Input: part model. Units: mm. Frame: model coordinates. A direction names the side the tool comes from. Coordinates: 2 decimals unless noted, no trailing zeros. Loops run counter-clockwise (first coordinate to the right, second up) from the corner with the lowest first, then second, coordinate; pieces in that order, holes last. Notation, with made-up numbers: (64, -15.5) -> (97, -15.5) arc R22 ccw to (97, 23.5) -> close; hole circle Ø9 at (70, 56.5). An arc over 180 degrees is marked (long way). Answer as a JSON object with one key per item and string values.
from build123d import *

# Parameters (mm, degrees)
PAD004_DEPTH    = 25
SKETCH032_W     = 8
SKETCH032_H     = 19
PAD005_DEPTH    = 5
SKETCH033_R     = 1.25
POCKET006_DEPTH = 12.001
FILLET_R        = 2.49
CHAMFER009_SIZE = 0.3
CHAMFER010_SIZE = 0.5


with BuildPart() as part:
    # Sketch031 → Pad004 (new body)
    with BuildSketch(Plane.XZ):
        with BuildLine():
            Line((-7.5, -5), (-7.5, -6.5))
            ThreePointArc((-7.5, -6.5), (-7.353553, -6.853553), (-7, -7))
            Line((-7, -7), (7, -7))
            ThreePointArc((7, -7), (7.353553, -6.853553), (7.5, -6.5))
            Line((7.5, -6.5), (7.5, -5))
            Line((7.5, -5), (12, -5))
            Line((12, -5), (13, -6))
            Line((13, -6), (13, -11))
            Line((13, -11), (12, -12))
            Line((12, -12), (-12, -12))
            Line((-12, -12), (-13, -11))
            Line((-13, -11), (-13, -6))
            Line((-13, -6), (-12, -5))
            Line((-12, -5), (-7.5, -5))
        make_face()
    extrude(amount=PAD004_DEPTH)

    # Sketch032 → Pad005 (join)
    with BuildSketch(Plane.XZ):
        with Locations((0, -2.5)):
            Rectangle(SKETCH032_W, SKETCH032_H)
    extrude(amount=-PAD005_DEPTH)

    # Sketch033 → Pocket006 (cut, through all)
    with BuildSketch(Plane.XY):
        with Locations((0, -15)):
            Circle(SKETCH033_R)
    extrude(amount=-POCKET006_DEPTH, mode=Mode.SUBTRACT)

    # Fillet
    fillet_edges = [part.edges().sort_by_distance(p)[0] for p in [
        (4, 0, -9.5),
        (-4, 0, -9.5),
        (-4, 5, -2.5),
        (4, 5, -2.5),
    ]]
    fillet(fillet_edges, radius=FILLET_R)

    # Chamfer009
    chamfer009_edges = [part.edges().sort_by_distance(p)[0] for p in [
        (-1.25, -15, -7),
        (-1.25, -15, -12),
    ]]
    chamfer(chamfer009_edges, length=CHAMFER009_SIZE)

    # Chamfer010
    chamfer010_edges = [part.edges().sort_by_distance(p)[0] for p in [
        (-7.5, -25, -5.75),
        (-7.353553, -25, -6.853553),
        (0, -25, -7),
        (7.353553, -25, -6.853553),
        (7.5, -25, -5.75),
        (9.75, -25, -5),
        (12.5, -25, -5.5),
        (13, -25, -8.5),
        (12.5, -25, -11.5),
        (0, -25, -12),
        (-12.5, -25, -11.5),
        (-13, -25, -8.5),
        (-12.5, -25, -5.5),
        (-9.75, -25, -5),
        (-4, 1.255, 7),
        (-3.270696, 4.270696, 7),
        (0, 0, 7),
        (0, 5, 7),
        (4, 1.255, 7),
        (3.270696, 4.270696, 7),
        (13, 0, -8.5),
        (12.5, 0, -5.5),
        (12.5, 0, -11.5),
        (9.75, 0, -5),
        (-9.75, 0, -5),
        (-12.5, 0, -5.5),
        (-13, 0, -8.5),
        (-12.5, 0, -11.5),
        (0, 5, -12),
    ]]
    chamfer(chamfer010_edges, length=CHAMFER010_SIZE)


with BuildPart() as part_1:
    # Body007 placement: moved
    add(part.part.moved(Location((0, 55, 0))))


solid = part_1.part
1. Section query D-D (x = -10.5). Return loops of the section in (y, z).
Reply:
{"outline": "(30, -11.5) -> (30.5, -12) -> (54.5, -12) -> (55, -11.5) -> (55, -5.5) -> (54.5, -5) -> (30.5, -5) -> (30, -5.5) -> close"}
2. Section query C-C (z = 3). Return loops of the section in (x, y).
Reply:
{"outline": "(-4, 55) -> (4, 55) -> (4, 57.51) arc R2.49 ccw to (1.51, 60) -> (-1.51, 60) arc R2.49 ccw to (-4, 57.51) -> close"}
3. Section query A-A (y = 40). Return loops of the section in (x, z), plus the area to 3 significant figures.
Reply:
{"outline": "(-13, -11) -> (-12, -12) -> (-1.55, -12) -> (-1.25, -11.7) -> (-1.25, -7.3) -> (-1.55, -7) -> (-7, -7) arc R0.5 cw to (-7.5, -6.5) -> (-7.5, -5) -> (-12, -5) -> (-13, -6) -> close; (1.25, -11.7) -> (1.55, -12) -> (12, -12) -> (13, -11) -> (13, -6) -> (12, -5) -> (7.5, -5) -> (7.5, -6.5) arc R0.5 cw to (7, -7) -> (1.55, -7) -> (1.25, -7.3) -> close", "area": "137 mm2"}
4. Pin query (flat end, axial travel): P1, Ø1.3, axis at x = 9, y = 37.5, coming from the +Z side; P2, Ø4, axis at y = 55, z = -1, coming from the +X side; P3, Ø1.2, axis at y = 37.5, z = -5.5, coming from the -X side; P4, Ø4, axis at x = 0, z = -0.5, coming from the -Y side. Return the tip coordinate at first contact, or that it passes through.
Reply:
{"P1": "stops at z = -5", "P2": "stops at x = 4", "P3": "stops at x = -13", "P4": "stops at y = 55"}
5. Section query B-B (x = 0). Return loops of the section in (y, z).
Reply:
{"outline": "(30, -11.5) -> (30.5, -12) -> (38.45, -12) -> (38.75, -11.7) -> (38.75, -7.3) -> (38.45, -7) -> (30.5, -7) -> (30, -7.5) -> close; (41.25, -11.7) -> (41.55, -12) -> (59.5, -12) -> (60, -11.5) -> (60, 6.5) -> (59.5, 7) -> (55.5, 7) -> (55, 6.5) -> (55, -7) -> (41.55, -7) -> (41.25, -7.3) -> close"}
6. Access query for faces 4 (the face through (-7.5, 43, -6)), 5 (the face through (7.483, 30.309, -6.994)), 6 (the face through (-9, 55, -8)). Directions: +Z, -Z, +X, -X, +Y, -Y. A direction counts if a zero-diameter tool reaches every point of the face in a straight line with its end or side. Return the directions, or none.
Reply:
{"face 4": "+Z, +Y, -Y", "face 5": "+Z, -Y", "face 6": "+Z, -Z, -X, +Y"}
7. Line query: line 1 along Y through (x, z) = (0, -9.75); line 2 along Y through (x, z) = (0.5, 5); line 3 along Z through (x, y) = (-2.5, 51). Output: solid intervals per line, ascending.
Reply:
{"line 1": "y = 30 to 38.75, 41.25 to 60", "line 2": "y = 55 to 60", "line 3": "z = -12 to -7"}
8. Mould query, pull axis X, two halves, no side actions, for faces 1 (the face through (7.5, 43, -6)), 2 (the face through (-12.33, 54.75, -5.68)), 3 (the face through (4, 56, -1)). Classes: pulls with the +X half, pulls with the -X half, needs draft (parallel to the pull), parting line crosses it, or undercut.
Reply:
{"face 1": "undercut", "face 2": "pulls with the -X half", "face 3": "pulls with the +X half"}
